Verification items for the finished model (mm, model axes). Give positions to 0.01 mm unless a question says otherwise; leave off trailing zeros. Order: outer loops, then holes, each group sorted by start corner. A loop starts at its lowest first (then second) coordinate and runs counter-clockwise, first axis right, second up.
(1) Scan lines: L1, parallel to Y at x = 40, z = 11; L2, parallel to Z at x = -8.5, y = -21.5; L3, parallel to Y at x = 29.5, z = 6.75. Record each from-to range of solid material in increasing order.
(2) Gauge pin test, flat ends, axial feed: pin 1 (6.5 mm diameter, centred on y = -15, z = 5.5, fed in from -X); pin 2 (0.9 mm diameter, centred on y = -0.5, z = 10.5, fed in from +X); pin 3 (1 mm diameter, centred on x = 16, y = 19, fed in from -Z); pin 4 (5 mm diameter, centred on x = -77, z = 8, fed in from +Y). Record the tip position at first contact, or that the pin passes through.
(3) Sectioned sample at C-C on y = -27.5. Record the cut outline in (x, z).
(4) Sectioned sample at A-A on x = 38. Record the cut outline in (y, z).
(5) Sectioned sample at B-B on y = 0. Record the cut outline in (x, z).
(6) Sectioned sample at D-D on y = 14.5. Record the cut outline in (x, z), plus the area to 3 significant figures.
```python
from build123d import *

# Parameters (mm, degrees)
PAD_DEPTH       = 9
POCKET_DEPTH    = 6
SKETCH002_W     = 26.5
SKETCH002_H     = 35
POCKET001_DEPTH = 6
SKETCH003_W     = 127
SKETCH003_H     = 6
PAD001_DEPTH    = 3


with BuildPart() as part:
    # Sketch → Pad (new body)
    with BuildSketch(Plane.XY):
        with BuildLine():
            ThreePointArc((-65, 41), (-106, 0), (-65, -41))
            Line((-65, -41), (65, -41))
            ThreePointArc((65, -41), (106, 0), (65, 41))
            Line((-65, 41), (65, 41))
        make_face()
    extrude(amount=PAD_DEPTH)

    # Sketch001 (on Face6 of Pad) → Pocket (cut)
    with BuildSketch(Plane.XY.offset(9)):
        with BuildLine():
            ThreePointArc((-62.5, 6), (-68.5, 0), (-62.5, -6))
            Line((-62.5, -6), (62.5, -6))
            ThreePointArc((62.5, -6), (68.5, 0), (62.5, 6))
            Line((-62.5, 6), (62.5, 6))
        make_face()
    extrude(amount=-POCKET_DEPTH, mode=Mode.SUBTRACT)

    # Sketch002 (on Face5 of Pocket) → Pocket001 (cut)
    with BuildSketch(Plane.XY.offset(9)):
        with Locations((0, -23.5)):
            Rectangle(SKETCH002_W, SKETCH002_H)
    extrude(amount=-POCKET001_DEPTH, mode=Mode.SUBTRACT)

    # Sketch003 (on Face5 of Pocket001) → Pad001 (join)
    with BuildSketch(Plane.XY.offset(9)):
        with BuildLine():
            ThreePointArc((-65, 41), (-106, 0), (-65, -41))
            Line((-65, -41), (65, -41))
            ThreePointArc((65, -41), (106, 0), (65, 41))
            Line((-65, 41), (65, 41))
        make_face()
        Rectangle(SKETCH003_W, SKETCH003_H, mode=Mode.SUBTRACT)
    extrude(amount=PAD001_DEPTH)


solid = part.part
```
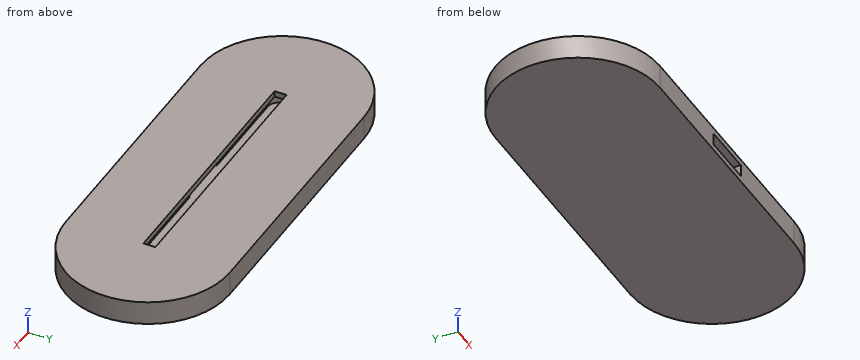
Ans:
1. L1: y = -41 to -3, 3 to 41
1. L2: z = 0 to 3, 9 to 12
1. L3: y = -41 to -6, 6 to 41
2. pin 1: stops at x = -104.28
2. pin 2: stops at x = 106
2. pin 3: stops at z = 0
2. pin 4: stops at y = 39.88
3. outline: (-95.41, 0) - (95.41, 0) - (95.41, 12) - (-95.41, 12) - close; hole (-13.25, 3) - (13.25, 3) - (13.25, 9) - (-13.25, 9) - close
4. outline: (-41, 0) - (41, 0) - (41, 12) - (3, 12) - (3, 9) - (6, 9) - (6, 3) - (-6, 3) - (-6, 9) - (-3, 9) - (-3, 12) - (-41, 12) - close
5. outline: (-106, 0) - (106, 0) - (106, 12) - (63.5, 12) - (63.5, 9) - (68.5, 9) - (68.5, 3) - (-68.5, 3) - (-68.5, 9) - (-63.5, 9) - (-63.5, 12) - (-106, 12) - close
6. outline: (-103.35, 0) - (103.35, 0) - (103.35, 12) - (-103.35, 12) - close
6. area: 2,480 mm2
